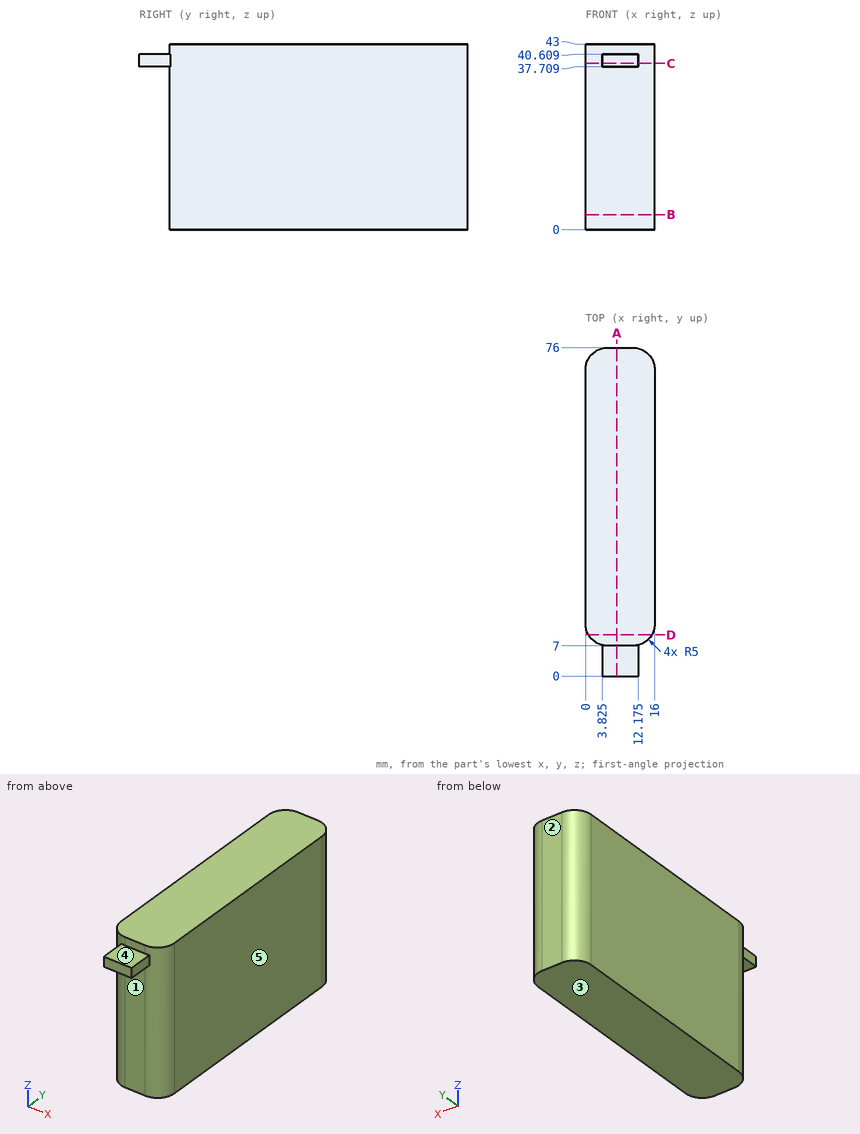
Geometry: see drawing. Coordinates: mm, zero at the bounding-box minimum. A direction names the side the tool comes from. Give positions to 0.01 mm unless a question says otherwise; leave off trailing zeros. Loops run counter-clockwise (first coordinate to the right, second up) from the corner with the lowest first, then second, coordinate; pieces in that order, holes last. Notation, with made-up numbers: (-9.75, -2) - (25.25, -2) arc R33 ccw to (25.25, 34) - close; hole circle Ø8 at (78, 74.5). An arc over 180 degrees is marked (long way). Answer as CSV lines item,"result". Start each with the question number.
1. Section C-C, the plane z = 38.5. Return loops of the section in (x, y) (1 decimal).
2. Draft query along Z for the marked faces 3, 4 and 5. Return one class per face: released by +Z, released by -Z, zero draft, split by the parting line, or undercut.
3. Pin query (flat end, axial travel): P1, Ø2, axis at x = 8.5, y = 4.5, coming from the -Z side; P2, Ø3, axis at y = 3, z = 40, coming from the -X side (1 decimal); P3, Ø8, axis at x = 8, z = 5.5, coming from the -Y side; P4, Ø8, axis at x = 9.5, y = 5, coming from the +Z side. Return the tip coordinate at first contact, or that it passes through.
4. Section A-A, the plane x = 7.25. Return loops of the section in (y, z).
5. Reachability of the marked faces 1 and 2 from +Z, -Z, +X, -X, +Y, -Y: full face, straight path, thin tool, end or side. Return the list, or none.
6. Ray query, L1, parallel to Y at x = 8.25, z = 22.5; L2, parallel to Y at x = 3.75, z = 13; L3, parallel to X at y = 11, z = 15.5. Return the intervals inside material, ascending.
7. Section B-B, the plane z = 3.5. Return loops of the section in (x, y).
8. Section D-D, the plane y = 9.5. Return loops of the section in (x, z).
Answers:
1,outline,"(0, 12) arc R5 ccw to (3.8, 7.1) - (3.8, 0) - (12.2, 0) - (12.2, 7.1) arc R5 ccw to (16, 12) - (16, 71) arc R5 ccw to (11, 76) - (5, 76) arc R5 ccw to (0, 71) - close"
2,face 3,"released by -Z"
2,face 4,"released by +Z"
2,face 5,"zero draft"
3,P1,"stops at z = 37.71"
3,P2,"stops at x = 3.8"
3,P3,"stops at y = 7"
3,P4,"stops at z = 43"
4,outline,"(0, 37.71) - (7, 37.71) - (7, 0) - (76, 0) - (76, 43) - (7, 43) - (7, 40.61) - (0, 40.61) - close"
5,face 1,"-Z, +X, -X, -Y"
5,face 2,"+Z, -Z, +X, -X, +Y"
6,L1,"y = 7 to 76"
6,L2,"y = 7.16 to 75.84"
6,L3,"x = 0.1 to 15.9"
7,outline,"(0, 12) arc R5 ccw to (5, 7) - (11, 7) arc R5 ccw to (16, 12) - (16, 71) arc R5 ccw to (11, 76) - (5, 76) arc R5 ccw to (0, 71) - close"
8,outline,"(0.67, 0) - (15.33, 0) - (15.33, 43) - (0.67, 43) - close"
